from build123d import *

# Parameters (mm, degrees)
BOSS_EXTRUDE1_DEPTH = 20
SKETCH2_W           = 20
SKETCH2_H           = 20
CUT_EXTRUDE1_DEPTH  = 74.484692283


with BuildPart() as part:
    # Sketch1 → Boss-Extrude1 (new body)
    with BuildSketch(Plane.XY):
        Polygon((50, 0), (-50, 0), (-50, 30), (0, 50), (50, 30), align=None)
    extrude(amount=BOSS_EXTRUDE1_DEPTH)

    # Sketch2 → Cut-Extrude1 (cut, through all)
    with BuildSketch(Plane.XY.offset(20)):
        with Locations((0, 10)):
            Rectangle(SKETCH2_W, SKETCH2_H)
    extrude(amount=-CUT_EXTRUDE1_DEPTH, mode=Mode.SUBTRACT)


solid = part.part
The listing builds one solid part. Answer for the finished solid, in the listing's coordinates (mm). A direction names the side the tool comes from. Coordinates: 2 decimals unless noted, no trailing zeros. Order: outer loops, then holes, each group sorted by start corner. A loop starts at its lowest first (then second) coordinate and runs counter-clockwise, first axis right, second up.
Q1. A cutting plane is placed at C-C, the plane x = 19. Write down the section's boundary in (y, z).
Q2. A cutting plane is placed at A-A, the plane y = 13.5. Write down the section's boundary in (x, z).
Q3. Given P1, Ø6, axis at x = 3, z = 6, coming from the -Y side; P2, Ø6, axis at y = 33.5, z = 11, coming from the -X side; P3, Ø12, axis at x = -38, z = 10.5, coming from the +Y side, each flat-ended and moving along its own axis, determine where each tip first touches the part or whether it passes through.
Q4. Which of the six approach directions +Z, -Z, +X, -X, +Y, -Y give full straight-line access (tool end or side, diameter ignored) to faces 1 (the face through (-50, 15, 10)), 2 (the face through (0, 20, 10))?
Q5. For a pull along X with two mould halves and no side action, classify faces 3 (the face through (-25, 40, 10)), 4 (the face through (1, 25, 20)), 5 (the face through (50, 15, 10)), 6 (the face through (10, 10, 10)) as pulls with the +X half, pulls with the -X half, needs draft (parallel to the pull), parting line crosses it, or undercut.
Q6. A cutting plane is placed at B-B, the plane z = 18. Write down the section's boundary in (x, y).
Q7. Consider line 1 (X direction, y = 9, z = 7.75); line 2 (Y direction, x = -41, z = 13.25); line 3 (Y direction, x = 21, z = 6). Determine where each line is inside the solid, lowest interval first.
Q8. A cutting plane is placed at D-D, the plane y = 46.5. Write down the section's boundary in (x, z), and give its area (3 significant figures).
Answers follow:
1. outline: (0, 0) - (42.4, 0) - (42.4, 20) - (0, 20) - close
2. outline: (-50, 0) - (-10, 0) - (-10, 20) - (-50, 20) - close; (10, 0) - (50, 0) - (50, 20) - (10, 20) - close
3. P1: stops at y = 20
3. P2: stops at x = -48.75
3. P3: stops at y = 37.2
4. face 1: +Z, -Z, -X, +Y, -Y
4. face 2: +Z, -Z, -Y
5. face 3: pulls with the -X half
5. face 4: needs draft
5. face 5: pulls with the +X half
5. face 6: undercut
6. outline: (-50, 0) - (-10, 0) - (-10, 20) - (10, 20) - (10, 0) - (50, 0) - (50, 30) - (0, 50) - (-50, 30) - close
7. line 1: x = -50 to -10, 10 to 50
7. line 2: y = 0 to 33.6
7. line 3: y = 0 to 41.6
8. outline: (-8.75, 0) - (8.75, 0) - (8.75, 20) - (-8.75, 20) - close
8. area: 350 mm2
